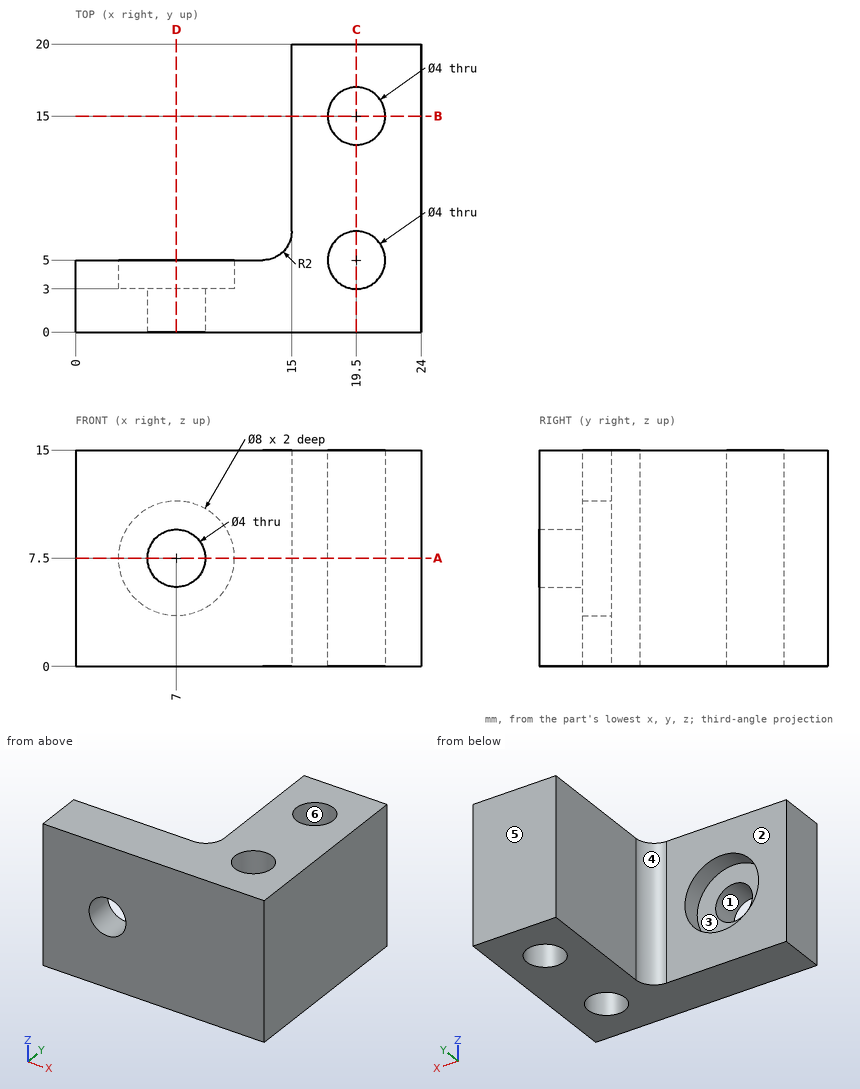
Check sheet for the drawn part. Datum: minimum x, y, z corner. Units: mm. A direction names the side the tool comes from. Round coordinates to 2 decimals unless told otherwise and drop trailing zeros. Order: outer loops, then holes, each group sorted by start corner. A loop starts at its lowest first (then second) coordinate and runs counter-clockwise, first axis right, second up.
1) Go/stop test with flat-tipped pins: pin 1 Ø3 at (y, z) = (10.5, 3.5) entering from -X; pin 2 Ø4 at (x, z) = (9, 5) entering from +Y. Record where each tip stops, or that it passes through.
2) Section check A-A (z = 7.5). Record the boundary of the cut face in (x, y).
3) Tool access check on the marked faces 1, 2 and 3. Record the directions out of +Z, -Z, +X, -X, +Y, -Y that give a thin tool (end or side, any length) a straight path to the whole face; none if there is none.
4) Mould release check, pull along X, two halves, no side actions. Record for the marked faces 4, 5 and 6: +X half, -X half, draft (parallel to the pull), parting line (faces both ways), or undercut.
5) Section check B-B (y = 15). Record the boundary of the cut face in (x, z), and give its area (3 significant figures).
6) Section check D-D (x = 7). Record the boundary of the cut face in (y, z).
7) Section check C-C (x = 19.5). Record the boundary of the cut face in (y, z).
8) Scan lines: line 1 (Y direction, x = 19.5, z = 8); line 2 (X direction, y = 0.8, z = 7.5); line 3 (X direction, y = 3.25, z = 6). Record each from-to range of solid material in increasing order.
Result:
1. pin 1: stops at x = 15
1. pin 2: stops at y = 5
2. outline: (0, 0) - (5, 0) - (5, 3) - (3, 3) - (3, 5) - (0, 5) - close; (9, 0) - (24, 0) - (24, 20) - (15, 20) - (15, 7) arc R2 cw to (13, 5) - (11, 5) - (11, 3) - (9, 3) - close; hole circle Ø4 at (19.5, 5); hole circle Ø4 at (19.5, 15)
3. face 1: +Y, -Y
3. face 2: +Z, -Z, -X, +Y
3. face 3: +Y
4. face 4: -X half
4. face 5: draft
4. face 6: undercut
5. outline: (15, 0) - (17.5, 0) - (17.5, 15) - (15, 15) - close; (21.5, 0) - (24, 0) - (24, 15) - (21.5, 15) - close
5. area: 75.0 mm2
6. outline: (0, 0) - (5, 0) - (5, 3.5) - (3, 3.5) - (3, 5.5) - (0, 5.5) - close; (0, 9.5) - (3, 9.5) - (3, 11.5) - (5, 11.5) - (5, 15) - (0, 15) - close
7. outline: (0, 0) - (3, 0) - (3, 15) - (0, 15) - close; (7, 0) - (13, 0) - (13, 15) - (7, 15) - close; (17, 0) - (20, 0) - (20, 15) - (17, 15) - close
8. line 1: y = 0 to 3, 7 to 13, 17 to 20
8. line 2: x = 0 to 5, 9 to 24
8. line 3: x = 0 to 3.29, 10.71 to 18.53, 20.47 to 24
